from build123d import *

# Parameters (mm, degrees)
SKETCH1_W           = 38.1
SKETCH1_H           = 76.2
BOSS_EXTRUDE1_DEPTH = 6.35
SKETCH2_R           = 4.2418
SKETCH2_R_2         = 3.302
CUT_EXTRUDE1_DEPTH  = 6.35
CHAMFER1_SIZE       = 1.27
SKETCH4_R           = 5.588
CUT_EXTRUDE2_DEPTH  = 2.54
SKETCH3_R           = 7.112
CUT_EXTRUDE3_DEPTH  = 3.81


with BuildPart() as part:
    # Sketch1 → Boss-Extrude1 (new body)
    with BuildSketch(Plane.XY):
        with Locations((31.774534541, 118.99557006)):
            Rectangle(SKETCH1_W, SKETCH1_H)
    extrude(amount=BOSS_EXTRUDE1_DEPTH)

    # Sketch2 → Cut-Extrude1 (cut)
    with BuildSketch(Plane.XY.offset(6.35)):
        with Locations((31.774534541, 138.04557006)):
            Circle(SKETCH2_R)
        with Locations((31.774534541, 99.94557006)):
            Circle(SKETCH2_R_2)
    extrude(amount=-CUT_EXTRUDE1_DEPTH, mode=Mode.SUBTRACT)

    # Chamfer1
    chamfer1_edges = [part.edges().sort_by_distance(p)[0] for p in [
        (50.824534541, 118.99557006, 6.35),
        (31.774534541, 157.09557006, 6.35),
        (12.724534541, 118.99557006, 6.35),
        (31.774534541, 80.89557006, 6.35),
    ]]
    chamfer(chamfer1_edges, length=CHAMFER1_SIZE)

    # Sketch4 → Cut-Extrude2 (cut)
    with BuildSketch(Plane.XY.offset(6.35)):
        with Locations((31.774534541, 99.94557006)):
            Circle(SKETCH4_R)
    extrude(amount=-CUT_EXTRUDE2_DEPTH, mode=Mode.SUBTRACT)

    # Sketch3 → Cut-Extrude3 (cut)
    with BuildSketch(Plane.XY.offset(6.35)):
        with Locations((31.774534541, 138.04557006)):
            Circle(SKETCH3_R)
    extrude(amount=-CUT_EXTRUDE3_DEPTH, mode=Mode.SUBTRACT)


solid = part.part
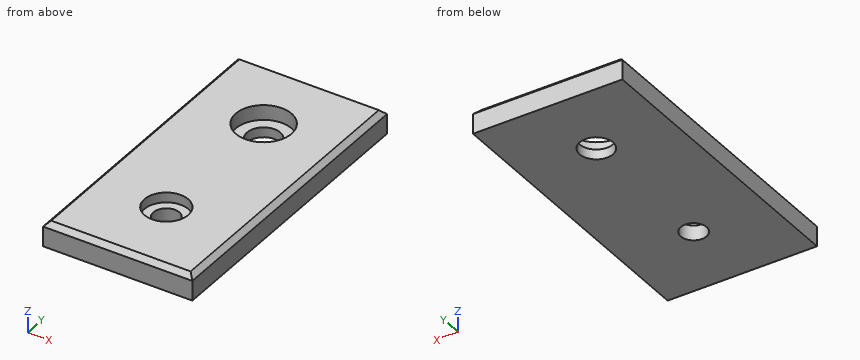
Verification items for the finished model (mm, model axes). Give positions to 0.01 mm unless a question says otherwise; leave off trailing zeros. Write each loop counter-clockwise with the first axis right and the second up, starting at its lowest first coordinate (ties: lowest second). Pieces come first, ordered by that corner, then holes.
(1) Cross-section at A-A (y = 101). Enter the section's corners in (x, z), plus the area to 3 significant figures.
(2) Gauge pin test, flat end, axial feed: pin 1 (4.5 mm diameter, centred on x = 34, y = 136, fed in from +Z). Record the tip position at first contact, or that the pin passes through.
(3) Material ranges on line 1 (Y direction, x = 32.5, z = 0.75); line 2 (Y direction, x = 31, z = 3.25); line 3 (Z direction, x = 28, y = 100.5), recorded low to high.
(4) Cross-section at B-B (z = 1.5). Enter the section's corners in (x, y).
Worked out:
1. outline: (12.72, 0) - (28.65, 0) - (28.65, 3.81) - (26.29, 3.81) - (26.29, 6.35) - (13.99, 6.35) - (12.72, 5.08) - close; (34.9, 0) - (50.82, 0) - (50.82, 5.08) - (49.55, 6.35) - (37.26, 6.35) - (37.26, 3.81) - (34.9, 3.81) - close
1. area: 189 mm2
2. pin 1: stops at z = 2.54
3. line 1: y = 80.9 to 96.72, 103.17 to 133.87, 142.22 to 157.1
3. line 2: y = 80.9 to 96.74, 103.16 to 130.98, 145.12 to 157.1
3. line 3: z = 0 to 3.81
4. outline: (12.72, 80.9) - (50.82, 80.9) - (50.82, 157.1) - (12.72, 157.1) - close; hole circle Ø8.48 at (31.77, 138.05); hole circle Ø6.6 at (31.77, 99.95)
